```python
from build123d import *

# Parameters (mm, degrees)
F0_W     = 33
F0_H     = 17.8
F1_DEPTH = 1.6
F2_R     = 0.5
F3_W     = 6
F3_H     = 6
F4_DEPTH = 1
F5_W     = 24
F5_H     = 1.5
F6_DEPTH = 2


with BuildPart() as f1:
    # F0 (on Top) → F1 (new body)
    with BuildSketch(Plane.XY):
        with Locations((2.53072, -1.123066)):
            Rectangle(F0_W, F0_H)
    extrude(amount=F1_DEPTH)

    # F2
    f2_edges = [f1.edges().sort_by_distance(p)[0] for p in [
        (19.03072, -10.023066, 0.8),
        (-13.96928, -10.023066, 0.8),
        (19.03072, 7.776934, 0.8),
        (-13.96928, 7.776934, 0.8),
    ]]
    fillet(f2_edges, radius=F2_R)

    # F3 (on face) → F4 (join)
    with BuildSketch(Plane.XY.offset(1.6)):
        with Locations((-3, 0.677927)):
            Rectangle(F3_W, F3_H)
    extrude(amount=F4_DEPTH)

    # F5 (on face) → F6 (join)
    with BuildSketch(Plane(origin=(0, 0, 0), x_dir=(1, 0, 0), z_dir=(0, 0, -1))):
        with Locations((3.64614, 7.426964)):
            Rectangle(F5_W, F5_H)
        with Locations((3.64614, -5.180832)):
            Rectangle(F5_W, F5_H)
    extrude(amount=F6_DEPTH)


solid = f1.part
```
CAD build for the part. Positions are in the model's coordinates, mm. A direction names the side the tool comes from. Round coordinates to 2 decimals unless told otherwise and drop trailing zeros. Write each loop counter-clockwise with the first axis right and the second up, starting at its lowest first coordinate (ties: lowest second). Pieces come first, ordered by that corner, then holes. Notation, with made-up numbers: (-2, 19.5) -> (31, 19.5) arc R28 ccw to (31, 54.5) -> close; hole circle Ø5 at (27.5, 35.5). An arc over 180 degrees is marked (long way). Answer in a Markdown table with one row per item. Add a question column.
Item 1: Saw through at A-A, the plane z = -1.55. Write the cut outline in (x, y), then the cut area to 3 significant figures.
Item 2: Saw through at C-C, the plane y = 0.5. Write the cut outline in (x, z), then the cut area to 3 significant figures.
Item 3: Drop flat-ended pins along their axis: pin 1 Ø0.6 at (x, z) = (2, -1) entering from -Y; pin 2 Ø1.5 at (x, y) = (13, 4) entering from -Z; pin 3 Ø0.8 at (y, z) = (5, -1) entering from +X; pin 4 Ø1 at (x, z) = (-1.5, -1) entering from +Y. Give the stop position or say it passes through.
Item 4: Which spindle directions (+Z, -Z, +X, -X, +Y, -Y) get a long thin tool onto all of the face, cutting with end or side? Do faces 1 (the face through (-8.354, -7, -1)), 2 (the face through (-6, 1, 2)), 3 (the face through (15.646, 5, -1)), 4 (the face through (-3, -2.322, 2)). Say none if no direction does.
Item 5: Saw through at B-B, the plane x = 9. Write the cut outline in (y, z).
Item 6: Mould opens along Y. For faces 5 (the face through (19.031, -1, 1)), 6 (the face through (3, 4.431, -1)), 7 (the face through (2, -1, 0)), 8 (the face through (-3, 3.678, 2)) say: pulls with the +Y half, pulls with the -Y half, needs draft (parallel to the pull), parting line crosses it, or undercut.
Item 7: Saw through at D-D, the plane x = -5. Write the cut outline in (y, z), then the cut area to 3 significant figures.
Item 8: Drill centre lines: line 1 (Y direction, x = 14, z = -1.4); line 2 (X direction, y = 1.25, z = 2.3); line 3 (Y direction, x = -4, z = 2.05). Where is each one in solid material? Low to high. Write a range as from..to.
Findings below:
| question | item | result |
|---|---|---|
| 1 | outline | (-8.35, -8.18) -> (15.65, -8.18) -> (15.65, -6.68) -> (-8.35, -6.68) -> close; (-8.35, 4.43) -> (15.65, 4.43) -> (15.65, 5.93) -> (-8.35, 5.93) -> close |
| 1 | area | 72.0 mm^2 |
| 2 | outline | (-13.97, 0) -> (19.03, 0) -> (19.03, 1.6) -> (0, 1.6) -> (0, 2.6) -> (-6, 2.6) -> (-6, 1.6) -> (-13.97, 1.6) -> close |
| 2 | area | 58.8 mm^2 |
| 3 | pin 1 | stops at y = -8.18 |
| 3 | pin 2 | stops at z = -2 |
| 3 | pin 3 | stops at x = 15.65 |
| 3 | pin 4 | stops at y = 5.93 |
| 4 | face 1 | -Z, -X, +Y, -Y |
| 4 | face 2 | +Z, -X, +Y, -Y |
| 4 | face 3 | -Z, +X, +Y, -Y |
| 4 | face 4 | +Z, +X, -X, -Y |
| 5 | outline | (-10.02, 0) -> (-8.18, 0) -> (-8.18, -2) -> (-6.68, -2) -> (-6.68, 0) -> (4.43, 0) -> (4.43, -2) -> (5.93, -2) -> (5.93, 0) -> (7.78, 0) -> (7.78, 1.6) -> (-10.02, 1.6) -> close |
| 6 | face 5 | needs draft |
| 6 | face 6 | undercut |
| 6 | face 7 | undercut |
| 6 | face 8 | pulls with the +Y half |
| 7 | outline | (-10.02, 0) -> (-8.18, 0) -> (-8.18, -2) -> (-6.68, -2) -> (-6.68, 0) -> (4.43, 0) -> (4.43, -2) -> (5.93, -2) -> (5.93, 0) -> (7.78, 0) -> (7.78, 1.6) -> (3.68, 1.6) -> (3.68, 2.6) -> (-2.32, 2.6) -> (-2.32, 1.6) -> (-10.02, 1.6) -> close |
| 7 | area | 40.5 mm^2 |
| 8 | line 1 | y = -8.18..-6.68, 4.43..5.93 |
| 8 | line 2 | x = -6..0 |
| 8 | line 3 | y = -2.32..3.68 |
